```python
from build123d import *

# Parameters (mm, degrees)
F0_W     = 76.2
F0_H     = 104.775
F0_R     = 1.5875
F0_R_2   = 8.334375
F1_DEPTH = 9.921875


# Not quite as in the source:
# - a length typed as a fraction of an inch, garbled in the dataset ("3 / 203.2 mm" for 3/8 in), is restored


with BuildPart() as f1:
    # F0 (on Front) → F1 (new body)
    with BuildSketch(Plane.XZ):
        with Locations((0, -3.96875)):
            Rectangle(F0_W, F0_H)
        with Locations((-25.003125, -23.8125)):
            Circle(F0_R, mode=Mode.SUBTRACT)
        with Locations((25.003125, -23.8125)):
            Circle(F0_R, mode=Mode.SUBTRACT)
        with Locations((-25.003125, 23.8125)):
            Circle(F0_R, mode=Mode.SUBTRACT)
        Circle(F0_R_2, mode=Mode.SUBTRACT)
        with Locations((25.003125, 23.8125)):
            Circle(F0_R, mode=Mode.SUBTRACT)
    extrude(amount=F1_DEPTH)


solid = f1.part
```
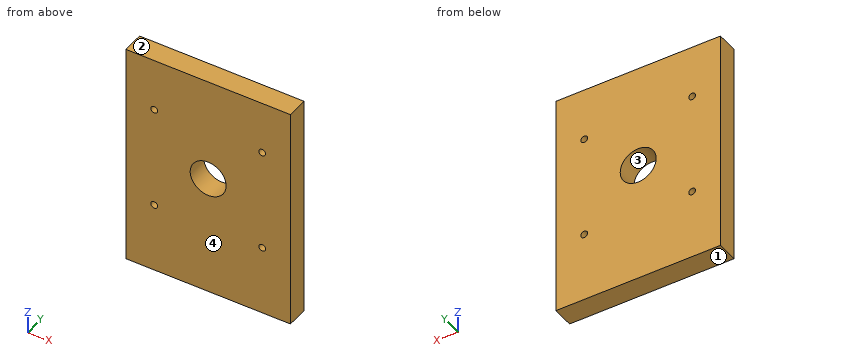
Work out the finished part from the listing and answer in its coordinate system (mm). Face numbers are marked on the shaded views. Give positions to 0.01 mm unless a question says otherwise; leave off trailing zeros. Order: outer loops, then holes, each group sorted by start corner. A loop starts at its lowest first (then second) coordinate and runs counter-clockwise, first axis right, second up.
1. The mould has two halves that part along Z. Classify the marked faces 1, 2, 3 and 4: released by +Z, released by -Z, zero draft, split by the parting line, or undercut.
Result sheet:
face 1: released by -Z
face 2: released by +Z
face 3: undercut
face 4: zero draft
2. Section A-A, the plane z = 0 is taken. Determine the outline of the cut face in (x, y), and give its area (3 significant figures).
Result sheet:
outline: (-38.1, -9.92) - (-8.33, -9.92) - (-8.33, 0) - (-38.1, 0) - close; (8.33, -9.92) - (38.1, -9.92) - (38.1, 0) - (8.33, 0) - close
area: 591 mm2
3. Section B-B, the plane x = 0 is taken. Determine the outline of the cut face in (y, z).
Result sheet:
outline: (-9.92, -56.36) - (0, -56.36) - (0, -8.33) - (-9.92, -8.33) - close; (-9.92, 8.33) - (0, 8.33) - (0, 48.42) - (-9.92, 48.42) - close
4. Straight lines are drawn through the part: L1, parallel to X at y = -6.5, z = 0.5; L2, parallel to X at y = -5.5, z = -1.5; L3, parallel to Z at x = -24.5, y = -1.25. For each, find the intervals that lie inside material, in ascending order.
Result sheet:
L1: x = -38.1 to -8.32, 8.32 to 38.1
L2: x = -38.1 to -8.2, 8.2 to 38.1
L3: z = -56.36 to -25.32, -22.31 to 22.31, 25.32 to 48.42
5. Section C-C, the plane y = -1.75 is taken. Determine the outline of the cut face in (x, z) (1 decimal), and give its area (3 significant figures).
Result sheet:
outline: (-38.1, -56.4) - (38.1, -56.4) - (38.1, 48.4) - (-38.1, 48.4) - close; hole circle Ø3.2 at (-25, -23.8); hole circle Ø3.2 at (-25, 23.8); hole circle Ø16.7 at (0, 0); hole circle Ø3.2 at (25, -23.8); hole circle Ø3.2 at (25, 23.8)
area: 7,730 mm2
